Check sheet for the modelled part. Datum: model origin and axes. Units: mm. Face numbers are marked on the shaded views. A direction names the side the tool comes from. Coordinates: 2 decimals unless noted, no trailing zeros. Loops run counter-clockwise (first coordinate to the right, second up) from the corner with the lowest first, then second, coordinate; pieces in that order, holes last. Notation, with made-up numbers: (85.25, 58) - (124.25, 58) arc R12 cw to (124.25, 69) - close; hole circle Ø2 at (20.25, 59). An arc over 180 degrees is marked (long way). Use a Markdown table: item, result. Add a question column.
1) Tool access check on the marked faces 1 and 2. Record the directions out of +Z, -Z, +X, -X, +Y, -Y that give a thin tool (end or side, any length) a straight path to the whole face; none if there is none.
2) Sectioned sample at B-B, the plane y = 8.5. Enter the section's corners in (x, z).
3) Sectioned sample at A-A, the plane z = 2.35. Enter the section's corners in (x, y), then the cut area to 3 significant figures.
4) Sectioned sample at C-C, the plane x = 2. Enter the section's corners in (y, z).
5) Go/stop test with flat-tipped pins: P1, Ø0.8, axis at y = -0.5, z = 2.5, coming from the +X side; P2, Ø5, axis at x = -8, y = 6, coming from the +Z side; P3, Ø0.5, axis at x = 2.5, z = 2.5, coming from the -Y side. Record where each tip stops, or that it passes through.
6) Sectioned sample at D-D, the plane y = -10.5. Enter the section's corners in (x, z).
7) Thickness scan on line 1 (Z direction, x = 4, y = -2.5); line 2 (Z direction, x = -11.75, y = 11.75); line 3 (X direction, y = 8, z = 0.75). Record the ranges inside material, lowest first.
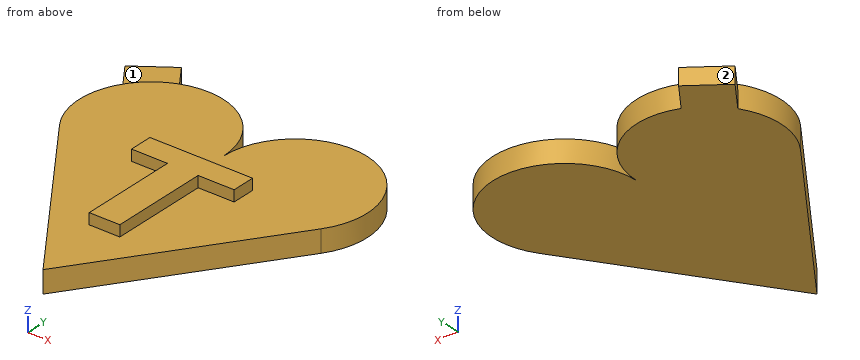
Autodesk Inventor part; units mm, degrees
ref_plane "YZ Plane" through (0, 0, 0) normal (1, 0, 0) x (0, 1, 0)
ref_plane "XZ Plane" through (0, 0, 0) normal (0, 1, 0) x (-1, 0, 0)
ref_plane "XY Plane" through (0, 0, 0) normal (0, 0, 1) x (1, 0, 0)
sketch "Sketch1" plane through (0, 0, 0) normal (0, 0, 1) x (1, 0, 0)
  line L0 (0, -14) -> (-11.8124, 2.7546)
  line L1 (0, -14) -> (11.8124, 2.7546)
  arc A0 (0, 6.5) -> (-11.8124, 2.7546) centre (-6.5, 6.5) ccw
  arc A1 (11.8124, 2.7546) -> (0, 6.5) centre (6.5, 6.5) ccw
  point P0 (0, 0)
extrude "Extrusion1" add sketch "Sketch1" along normal blind 2
sketch "Sketch6" plane through (0, 0, 0) normal (0, 0, -1) x (-1, 0, 0)
  line L0 (-11.8124, 2.7546) -> (0, -14)
  line L1 (11.8124, 2.7546) -> (0, -14)
  line L2 (0, -14) -> (0, -7)
  line L3 (-4.9352, -7) -> (4.9352, -7)
  line L4 (-1.3817, -7) -> (-1.3817, 1.9052)
  line L5 (-1.3817, 1.9052) -> (-4.6353, 1.9052)
  line L6 (-4.6353, 1.9052) -> (-4.6353, 4)
  line L7 (-4.6353, 4) -> (4.6353, 4)
  line L8 (4.6353, 4) -> (4.6353, 1.9052)
  line L9 (4.6353, 1.9052) -> (1.3817, 1.9052)
  line L10 (1.3817, 1.9052) -> (1.3817, -7)
  line L11 (1.3817, -7) -> (-1.3817, -7)
  point P0 (0, 0)
  dimension "d24" = 7
extrude "Extrusion5" add sketch "Sketch6" against normal blind 3 contours L4 L5 L6 L7 L8 L9 L10 L3
sketch "Sketch7" plane through (0, 0, 0) normal (0, 0, -1) x (-1, 0, 0)
  arc A0 (11.8124, 2.7546) -> (0, 6.5) centre (6.5, 6.5) ccw
  line L0 (10.6694, 15.1841) -> (8.8261, 12.5695)
  line L1 (13.9386, 12.8792) -> (10.6694, 15.1841)
  line L2 (11.9445, 10.0507) -> (13.9386, 12.8792)
  point P0 (0, 0)
extrude "Extrusion6" add sketch "Sketch7" against normal blind 1.5
properties part number "Gift - T"
Solved:
| question | item | result |
|---|---|---|
| 1 | face 1 | +Z, -X, +Y |
| 1 | face 2 | +Z, -Z, -X, +Y |
| 2 | outline | (-12.68, 0) - (-0.32, 0) - (-0.32, 2) - (-12.68, 2) - close; (0.32, 0) - (12.68, 0) - (12.68, 2) - (0.32, 2) - close |
| 3 | outline | (-4.64, 1.91) - (-1.38, 1.91) - (-1.38, -7) - (1.38, -7) - (1.38, 1.91) - (4.64, 1.91) - (4.64, 4) - (-4.64, 4) - close |
| 3 | area | 44.0 mm2 |
| 4 | outline | (-11.16, 0) - (11.19, 0) - (11.19, 2) - (4, 2) - (4, 3) - (1.91, 3) - (1.91, 2) - (-11.16, 2) - close |
| 5 | P1 | stops at x = 1.38 |
| 5 | P2 | stops at z = 2 |
| 5 | P3 | stops at y = 1.91 |
| 6 | outline | (-2.47, 0) - (2.47, 0) - (2.47, 2) - (-2.47, 2) - close |
| 7 | line 1 | z = 0 to 2 |
| 7 | line 2 | z = 0 to 1.5 |
| 7 | line 3 | x = -12.82 to -0.18, 0.18 to 12.82 |
